```python
from build123d import *

# Parameters (mm, degrees)
BOSS_EXTRUDE1_DEPTH      = 13
BOSS_EXTRUDE1_DEPTH_BACK = 13
CUT_EXTRUDE1_DEPTH       = 6.5
CUT_EXTRUDE1_DEPTH_BACK  = 6.5
CUT_EXTRUDE3_DEPTH       = 4.5
CUT_EXTRUDE3_DEPTH_BACK  = 4.5
SKETCH3_R                = 12
CUT_EXTRUDE4_DEPTH       = 10
CUT_EXTRUDE4_DEPTH_BACK  = 10
SKETCH4_R                = 4.25
SKETCH5_R                = 2
CUT_EXTRUDE5_DEPTH       = 47.828649116
SKETCH9_W                = 5.05
SKETCH9_H                = 13.520724833
CUT_EXTRUDE8_DEPTH       = 43.698622671
CUT_EXTRUDE9_DEPTH       = 42.532474067
FILLET1_R                = 4
CUT_EXTRUDE10_DEPTH      = 2.25


with BuildPart() as part:
    # Sketch1 → Boss-Extrude1 (new, two sides: drawn at the far end of the back side and taken through both)
    with BuildSketch(Plane.XY.offset(-BOSS_EXTRUDE1_DEPTH_BACK)):
        with BuildLine():
            Line((-1.754221061, 5.475875133), (-1.754221061, 37.575875133))
            Line((-1.754221061, 37.575875133), (10.245778939, 37.575875133))
            Line((10.245778939, 37.575875133), (10.245778939, -0.724124867))
            Line((10.245778939, -0.724124867), (2.875, -4.979646072))
            ThreePointArc((2.875, -4.979646072), (-5.257710269, -2.327870857), (-1.754221061, 5.475875133))
        make_face()
    extrude(amount=BOSS_EXTRUDE1_DEPTH + BOSS_EXTRUDE1_DEPTH_BACK)

    # Sketch2 → Cut-Extrude1 (cut, two sides: drawn at the far end of the back side and taken through both)
    with BuildSketch(Plane.XY.offset(-CUT_EXTRUDE1_DEPTH_BACK)):
        with BuildLine():
            Line((8.244357503, -1.879646072), (5.369357503, 3.1))
            ThreePointArc((5.369357503, 3.1), (2.300687806, 5.757328862), (-1.754221061, 5.946655234))
            Line((-1.754221061, 5.946655234), (-5.75, 5.946655234))
            Line((-5.75, 5.946655234), (-5.75, -5.75))
            Line((-5.75, -5.75), (8.244357503, -5.75))
            Line((8.244357503, -5.75), (8.244357503, -1.879646072))
        make_face()
    extrude(amount=CUT_EXTRUDE1_DEPTH + CUT_EXTRUDE1_DEPTH_BACK, mode=Mode.SUBTRACT)

    # Sketch3 → Cut-Extrude3 (cut, two sides: drawn at the far end of the back side and taken through both)
    with BuildSketch(Plane.XY.offset(-CUT_EXTRUDE3_DEPTH_BACK)):
        with Locations((0.245778939, 16.750875133)):
            Circle(SKETCH3_R)
    extrude(amount=CUT_EXTRUDE3_DEPTH + CUT_EXTRUDE3_DEPTH_BACK, mode=Mode.SUBTRACT)

    # Sketch4 → Cut-Extrude4 (cut, two sides: drawn at the far end of the back side and taken through both)
    with BuildSketch(Plane.XY.offset(-CUT_EXTRUDE4_DEPTH_BACK)):
        with Locations((0.245778939, 16.750875133)):
            Circle(SKETCH4_R)
    extrude(amount=CUT_EXTRUDE4_DEPTH + CUT_EXTRUDE4_DEPTH_BACK, mode=Mode.SUBTRACT)

    # Sketch5 → Cut-Extrude5 (cut, through all)
    with BuildSketch(Plane.XY.offset(13)):
        Circle(SKETCH5_R)
    extrude(amount=-CUT_EXTRUDE5_DEPTH, mode=Mode.SUBTRACT)

    # Sweep4: sweep along a path in Sketch8
    with BuildLine(Plane(origin=(0, 0, 4.5), x_dir=(-1, 0, 0), z_dir=(0, 0, -1))) as sweep4_path:
        CenterArc((-0.245778939, 16.750875133), 4.25, 0, 360)
    # 3DSketch3 → Sweep4 (sweep)
    with BuildSketch(Plane(origin=(4.495778939, 16.750875133, 4.5), x_dir=(1, 0, 0), z_dir=(0, 1, 0))):
        Polygon((0, 0), (2.8, 0), (1.75, 1.05), (0, 1.05), align=None)
    sweep4 = sweep(path=sweep4_path.line)

    # Mirror10: Sweep4 across plane
    add(sweep4.mirror(Plane.XY))

    # Sketch9 → Cut-Extrude8 (cut, through all)
    with BuildSketch(Plane(origin=(0, 0, 4.5), x_dir=(-1, 0, 0), z_dir=(0, 0, -1))):
        with Locations((4.279221061, 16.750875132)):
            Rectangle(SKETCH9_W, SKETCH9_H)
    extrude(amount=CUT_EXTRUDE8_DEPTH, mode=Mode.SUBTRACT)

    # Sketch10 → Cut-Extrude9 (cut, through all)
    with BuildSketch(Plane.ZY.offset(1.754221061)):
        with BuildLine():
            Line((-5.675, 32.750875133), (-5.675, 31.750875133))
            ThreePointArc((-5.675, 31.750875133), (-8, 29.425875133), (-10.325, 31.750875133))
            Line((-10.325, 31.750875133), (-10.325, 32.750875133))
            ThreePointArc((-10.325, 32.750875133), (-8, 35.075875133), (-5.675, 32.750875133))
        make_face()
        with BuildLine():
            Line((5.675, 32.750875133), (5.675, 31.750875133))
            ThreePointArc((5.675, 31.750875133), (8, 29.425875133), (10.325, 31.750875133))
            Line((10.325, 31.750875133), (10.325, 32.750875133))
            ThreePointArc((10.325, 32.750875133), (8, 35.075875133), (5.675, 32.750875133))
        make_face()
    extrude(amount=-CUT_EXTRUDE9_DEPTH, mode=Mode.SUBTRACT)

    # Fillet1
    fillet1_edges = [part.edges().sort_by_distance(p)[0] for p in [
        (4.245778939, 37.575875133, -13),
        (4.245778939, 37.575875133, 13),
    ]]
    fillet(fillet1_edges, radius=FILLET1_R)

    # Sketch11 → Cut-Extrude10 (cut)
    with BuildSketch(Plane.XY.offset(-6.5)):
        Polygon((0, 3.5), (-3.031088913, 1.75), (-3.031088913, -1.75), (0, -3.5), (3.031088913, -1.75), (3.031088913, 1.75), align=None)
    extrude(amount=-CUT_EXTRUDE10_DEPTH, mode=Mode.SUBTRACT)


solid = part.part
```
Could you check a few things on this model? Use its own coordinates, in mm. A direction names the side the tool comes from. Coordinates: 2 decimals unless noted, no trailing zeros. Write each loop counter-clockwise with the first axis right and the second up, starting at its lowest first coordinate (ties: lowest second). Pieces come first, ordered by that corner, then holes. Notation, with made-up numbers: M -34.5,55.25 L 3.5,55.25 A17 cw 3.5,75.25 Z; hole C 45.25,24 d7. An arc over 180 degrees is marked long. Answer as CSV lines item,"result". Start each with the question number.
1) For faces 4 (the flat face through (3.031, 0, -8)), 5 (the flat face through (4, 32, -5.675)), 6 (the cylindrical face through (0, -2, 10)), which set-ups out of +Z, -Z, +X, -X, +Y, -Y let a thin tool reach every point of the face, with its end or its side?
2) We'd pull the mould along Y, two halves only. Please class faces 1 (the flat face through (4, 37.576, 0)), 2 (the flat face through (4, 14, 13)), 3 (the cylindrical face through (4.162, 29.426, -7.949)): +Y half, -Y half, draft (parallel to the pull), parting line (faces both ways), or undercut.
3) Please list where these lines run through material, in increasing order: line 1 (Y direction, x = 0, z = 8); line 2 (Z direction, x = 4, y = -2); line 3 (Z direction, x = -1.5, y = 33.5). Write a range as from..to.
4) I want a section at A-A, the plane z = -8. Please give me the cut outline in (x, y) (3 decimals).
5) I want a section at D-D, the plane y = 0. Please give me the cut outline in (x, z), and give its area (3 significant figures).
6) I want a section at B-B, the plane x = -4.5. Please give me the cut outline in (y, z).
7) For P1, Ø5, axis at x = 0, y = 0, coming from the +Z side; P2, Ø2, axis at y = 9.5, z = 8.5, coming from the -X side, each with a flat end and sliding along its axis, tell me the tip position at first contact or that it passes through.
8) I want a section at C-C, the plane z = 2.25. Please give me the cut outline in (x, y).
Data:
1,face 4,"none"
1,face 5,"+X, -X"
1,face 6,"+Z, -Z"
2,face 1,"+Y half"
2,face 2,"draft"
2,face 3,"undercut"
3,line 1,"y = -5.75..-2, 2..12.51, 20.99..29.43, 35.08..37.58"
3,line 2,"z = -13..-6.5, 6.5..13"
3,line 3,"z = -13..-10.2, -5.8..5.8, 10.2..13"
4,outline,"M -1.754,5.476 A5.75 ccw long 2.875,-4.98 L 10.246,-0.724 L 10.246,29.426 L -1.754,29.426 L -1.754,20.501 A4.25 cw long -1.754,13.001 Z; M -1.754,35.076 L 10.246,35.076 L 10.246,37.576 L -1.754,37.576 Z; hole M -3.031,-1.75 L 0,-3.5 L 3.031,-1.75 L 3.031,1.75 L 0,3.5 L -3.031,1.75 Z"
5,outline,"M -5.75,-13 L -2,-13 L -2,-8.75 L -3.03,-8.75 L -3.03,-6.5 L -5.75,-6.5 Z; M -5.75,6.5 L -2,6.5 L -2,13 L -5.75,13 Z; M 2,-13 L 10.25,-13 L 10.25,13 L 2,13 L 2,6.5 L 7.16,6.5 L 7.16,-6.5 L 3.03,-6.5 L 3.03,-8.75 L 2,-8.75 Z"
5,area,"191 mm^2"
6,outline,"M -3.58,-13 L 3.58,-13 L 3.58,-6.5 L -3.58,-6.5 Z; M -3.58,6.5 L 3.58,6.5 L 3.58,13 L -3.58,13 Z"
7,P1,"stops at z = 13"
7,P2,"stops at x = -1.75"
8,outline,"M -1.75,28.58 A12 cw 10.25,23.38 L 10.25,37.58 L -1.75,37.58 Z; M 3.41,5.18 A6.2 cw 5.37,3.1 L 8.24,-1.88 L 10.25,-0.72 L 10.25,10.12 A12 cw Z"
